CAD build for the part. Positions are in the model's coordinates, mm. Face numbers are marked on the shaded views. A direction names the side the tool comes from. Coordinates: 2 decimals unless noted, no trailing zeros. Write each loop counter-clockwise with the first axis right and the second up, starting at its lowest first coordinate (ties: lowest second). Pieces come first, ordered by that corner, then holes. Notation, with made-up numbers: (-25, 50.5) -> (32, 50.5) arc R26 cw to (32, 89.5) -> close; hole circle Ø6 at (32.25, 64.5). An arc over 180 degrees is marked (long way). Answer as CSV lines item,"result".
Autodesk Inventor part; units mm, degrees
ref_plane "YZ Plane" through (0, 0, 0) normal (1, 0, 0) x (0, 1, 0)
ref_plane "XZ Plane" through (0, 0, 0) normal (0, 1, 0) x (-1, 0, 0)
ref_plane "XY Plane" through (0, 0, 0) normal (0, 0, 1) x (1, 0, 0)
sketch "Sketch1" plane through (0, 0, 0) normal (0, 0, 1) x (1, 0, 0)
  line L0 (0, -9.525) -> (0, 9.525) construction
  line L1 (7.9375, -9.525) -> (7.9375, 9.525)
  line L2 (-7.9375, 9.525) -> (-7.9375, -9.525)
  arc A0 (-7.9375, -9.525) -> (7.9375, -9.525) centre (0, -9.525) ccw
  arc A1 (7.9375, 9.525) -> (-7.9375, 9.525) centre (0, 9.525) ccw
  circle A2 centre (0, 10) radius 1.524
  circle A3 centre (0, -10) radius 1.524
  point P0 (0, 0)
  dimension "d0" = 15.875
  dimension "d1" = 3.048
  dimension "d2" = 3.048
  dimension "d3" = 20
  dimension "d4" = 10
  dimension "d5" = 9.525
extrude "Extrusion1" add sketch "Sketch1" along normal blind 5.08
sketch "Sketch2" plane through (0, 0, 5.08) normal (0, 0, 1) x (1, 0, 0)
  circle A0 centre (0, 10) radius 1.524
  circle A1 centre (0, -10) radius 1.524
  line L0 (0, 13.7395) -> (3.2385, 11.8697)
  line L1 (3.2385, 11.8697) -> (3.2385, 8.1302)
  line L2 (3.2385, 8.1302) -> (0, 6.2605)
  line L3 (0, 6.2605) -> (-3.2385, 8.1302)
  line L4 (-3.2385, 8.1302) -> (-3.2385, 11.8697)
  line L5 (-3.2385, 11.8697) -> (0, 13.7395)
  line L6 (0, -6.2605) -> (3.2385, -8.1302)
  line L7 (3.2385, -8.1302) -> (3.2385, -11.8697)
  line L8 (3.2385, -11.8697) -> (0, -13.7395)
  line L9 (0, -13.7395) -> (-3.2385, -11.8697)
  line L10 (-3.2385, -11.8697) -> (-3.2385, -8.1302)
  line L11 (-3.2385, -8.1302) -> (0, -6.2605)
  point P0 (0, 0)
  dimension "d8" = 6.477
extrude "Extrusion2" cut sketch "Sketch2" against normal blind 2.54
fillet "Fillet1" radius 3.81 4 edges at (0, -17.4625, 5.08) (7.9375, 0, 5.08) (0, 17.4625, 5.08) (-7.9375, 0, 5.08)
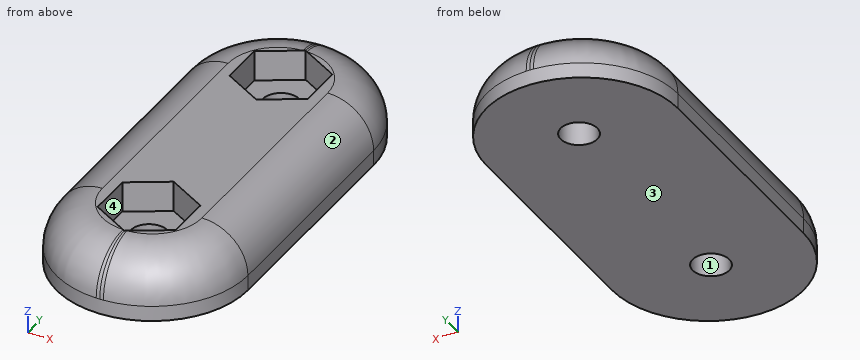
Item 1: 3-axis set-ups, long thin cutter, end or side, ignore diameter. For the marked faces 3 and 4: which of +Z, -Z, +X, -X, +Y, -Y reach the whole face in a straight line?
Answer below:
face 3,"-Z, +X, -X, +Y, -Y"
face 4,"+Z"
Item 2: Saw through at C-C on z = 4.2. State how many separate pieces and enclosed holes the cut face has, and give its area (3 significant figures).
Answer below:
separate pieces,"1"
enclosed holes,"2"
area,"313 mm2"
Item 3: Saw through at A-A on y = -2. Give the cut face in (x, z), and give its area (3 significant figures).
Answer below:
outline,"(-7.94, 0) -> (7.94, 0) -> (7.94, 1.27) arc R3.81 ccw to (4.13, 5.08) -> (-4.13, 5.08) arc R3.81 ccw to (-7.94, 1.27) -> close"
area,"74.4 mm2"
Item 4: Wall check: line 1 (Y direction, x = 0, z = 0.9); line 2 (Y direction, x = 0, z = 1.7); line 3 (Z direction, x = 1, y = -13). Give the ranges that are in metal, low to high. Write a range as from..to.
Answer below:
line 1,"y = -17.46..-11.52, -8.48..8.48, 11.52..17.46"
line 2,"y = -17.44..-11.52, -8.48..8.48, 11.52..17.44"
line 3,"z = 0..2.54"
Item 5: Saw through at B-B on z = 0.8. Give the cut face in (x, y) (1 decimal).
Answer below:
outline,"(-7.9, -9.5) arc R7.9 ccw to (7.9, -9.5) -> (7.9, 9.5) arc R7.9 ccw to (-7.9, 9.5) -> close; hole circle Ø3 at (0, -10); hole circle Ø3 at (0, 10)"
Item 6: Flat gauge pins, fed straight in: pin 1 (0.8 mm diameter, centred on y = 10.5, z = 3.5, fed in from -X); pin 2 (7 mm diameter, centred on x = 0, y = -10.5, fed in from +Z); pin 3 (1.5 mm diameter, centred on x = 0, z = 3, fed in from -Y); pin 4 (1.3 mm diameter, centred on y = -10, z = 3.5, fed in from -X). Where does each tip first touch, or does it go through?
Answer below:
pin 1,"stops at x = -7.41"
pin 2,"stops at z = 5.08"
pin 3,"stops at y = -17.33"
pin 4,"stops at x = -7.58"
Item 7: Two-plate mould, pull along Y, no slides. Class the marked faces 1 and 2: pulls with the +Y half, pulls with the -Y half, needs draft (parallel to the pull), parting line crosses it, or undercut.
Answer below:
face 1,"undercut"
face 2,"needs draft"
